CAD build for the part. Positions are in the model's coordinates, mm. Face numbers are marked on the shaded views. A direction names the side the tool comes from. Coordinates: 2 decimals unless noted, no trailing zeros. Loops run counter-clockwise (first coordinate to the right, second up) from the corner with the lowest first, then second, coordinate; pieces in that order, holes last. Notation, with made-up numbers: (-10, 36.25) -> (7, 36.25) arc R17 cw to (7, 42.25) -> close; hole circle Ø9 at (28.5, 46). An arc over 180 degrees is marked (long way). Answer as CSV lines item,"result". Start each with the question number.
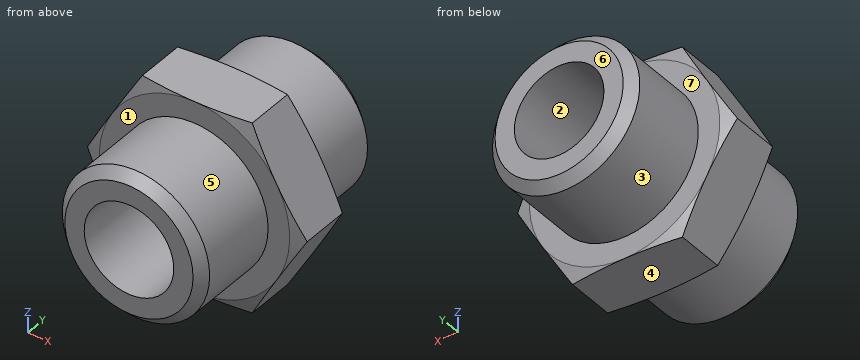
Autodesk Inventor part; units mm, degrees
ref_plane "IP1_XY" through (0, 0, 0) normal (0, 1, 0) x (1, 0, 0)
ref_plane "IP1_YZ" through (0, 0, 0) normal (1, 0, 0) x (0, 0, -1)
ref_plane "IP1_ZX" through (0, 0, 0) normal (0, 0, -1) x (0, 1, 0)
sketch "Sketch_6" plane through (0, 0, 0) normal (0, 0, 1) x (1, 0, 0)
  line L0 (0, 0) -> (0, 13)
  line L1 (0, 13) -> (8.5, 13)
  line L2 (8.5, 13) -> (10.2, 12.5445)
  line L3 (10.2, 12.5445) -> (10.2, 8.4555)
  line L4 (10.2, 8.4555) -> (8.5, 8)
  line L5 (8.5, 8) -> (6.5785, 8)
  line L6 (6.5785, 8) -> (6.5785, 0.856)
  line L7 (6.5785, 0.856) -> (5.7225, 0)
  line L8 (5.7225, 0) -> (0, 0)
  line L9 (0, 0) -> (0, 13)
revolve "Revolution1" add sketch "Sketch_6" angle 360 about axis through (0, 0, 0) along (0, -1, 0)
thread "Thread1"
sketch "Sketch_7" plane through (0, 0, 0) normal (0, 0, 1) x (1, 0, 0)
  line L0 (0, 13) -> (0, 21)
  line L1 (0, 21) -> (5.7225, 21)
  line L2 (5.7225, 21) -> (6.5785, 20.144)
  line L3 (6.5785, 20.144) -> (6.5785, 13)
  line L4 (6.5785, 13) -> (0, 13)
  line L5 (0, 13) -> (0, 21)
revolve "Revolution2" add sketch "Sketch_7" angle 360 about axis through (0, 13, 0) along (0, -1, 0)
thread "Thread2"
sketch "Sketch_10" plane through (0, 10.5, 0) normal (0, 1, 0) x (1, 0, 0)
  line L0 (-17, -17) -> (17, -17)
  line L1 (17, -17) -> (17, 17)
  line L2 (17, 17) -> (-17, 17)
  line L3 (-17, 17) -> (-17, -17)
  line L4 (-9.815, 0) -> (-4.9075, -8.5)
  line L5 (-4.9075, -8.5) -> (4.9075, -8.5)
  line L6 (4.9075, -8.5) -> (9.815, 0)
  line L7 (9.815, 0) -> (4.9075, 8.5)
  line L8 (4.9075, 8.5) -> (-4.9075, 8.5)
  line L9 (-4.9075, 8.5) -> (-9.815, 0)
extrude "Extrusion1" cut sketch "Sketch_10" along normal mid plane 12.6
sketch "Sketch4" plane through (0, 0, 0) normal (0, -1, 0) x (1, 0, 0)
  point P0 (0, 0)
hole "Hole1" at (0, 0, 0) direction (0, 1, 0) diameter 8 depth 21
ref_plane "IP1_XY" through (0, 0, 0) normal (0, 1, 0) x (1, 0, 0)
ref_plane "IP1_YZ" through (0, 0, 0) normal (1, 0, 0) x (0, 0, -1)
ref_plane "IP1_ZX" through (0, 0, 0) normal (0, 0, -1) x (0, 1, 0)
ref_plane "IP2_XY" through (0, 21, 0) normal (0, -1, 0) x (1, 0, 0)
ref_plane "IP2_YZ" through (0, 21, 0) normal (1, 0, 0) x (0, 0, 1)
ref_plane "IP2_ZX" through (0, 21, 0) normal (0, 0, 1) x (0, -1, 0)
ref_plane "RING1_XY" through (0, 8, 0) normal (0, 1, 0) x (1, 0, 0)
ref_plane "RING1_YZ" through (0, 8, 0) normal (1, 0, 0) x (0, 0, -1)
ref_plane "RING1_ZX" through (0, 8, 0) normal (0, 0, -1) x (0, 1, 0)
ref_plane "RING2_XY" through (0, 13, 0) normal (0, -1, 0) x (1, 0, 0)
ref_plane "RING2_YZ" through (0, 13, 0) normal (1, 0, 0) x (0, 0, 1)
ref_plane "RING2_ZX" through (0, 13, 0) normal (0, 0, 1) x (0, -1, 0)
properties part number "8030272 NPFC-D-2G14-M"
Q1. Pin check, flat tips, straight feed: pin 1 Ø1.5 at (y, z) = (3, 3) entering from +X; pin 2 Ø2 at (x, z) = (5, -5) entering from -Y; pin 3 Ø3 at (x, y) = (1.5, 2.5) entering from -Z. Stop position of each tip, or through.
Q2. Which spindle directions (+Z, -Z, +X, -X, +Y, -Y) get a long thin tool onto all of the face, cutting with end or side? Do the marked faces 5, 6 and 7. Say none if no direction does.
Q3. Probe probe 1 along Z at (x, y) = (0, 6.5); probe 2 along Z at (x, y) = (0, 9.5); probe 3 along Y at (x, z) = (-4, -6). List the from-to ranges inside material, lowest first. Write a range as from..to.
Q4. Two-plate mould, pull along Z, no slides. Class the marked faces 1, 2, 3 and 4: pulls with the +Z half, pulls with the -Z half, needs draft (parallel to the pull), parting line crosses it, or undercut.
Q5. Saw through at A-A (y = 3.75). List the corners of the cut face in (x, z), and give its area (3 significant figures).
Ans:
1,pin 1,"stops at x = 6.18"
1,pin 2,"stops at y = 0.35"
1,pin 3,"stops at z = -6.58"
2,face 5,"-Y"
2,face 6,"+Z, -Z, +X, -X, +Y"
2,face 7,"+Y"
3,probe 1,"z = -6.58..-4, 4..6.58"
3,probe 2,"z = -8.5..-4, 4..8.5"
3,probe 3,"y = 8..13"
4,face 1,"needs draft"
4,face 2,"undercut"
4,face 3,"parting line crosses it"
4,face 4,"pulls with the -Z half"
5,outline,"circle Ø13.16 at (0, 0); hole circle Ø8 at (0, 0)"
5,area,"85.7 mm²"
